```python
from build123d import *

# Parameters (mm, degrees)
CUT_EXTRUDE1_DEPTH = 1.8288


with BuildPart() as part:
    # Sketch1 → Revolve1 (revolve)
    with BuildSketch(Plane.XY, mode=Mode.PRIVATE) as revolve1_sk:
        with BuildLine():
            Line((0, 0), (76.9366, 0))
            Line((76.9366, 0), (76.9366, 2.413))
            Line((76.9366, 2.413), (0.7366, 2.413))
            Line((0.7366, 2.413), (0.7366, 4.5847))
            Line((0.7366, 4.5847), (0.3556, 4.5847))
            ThreePointArc((0.3556, 4.5847), (-0.901703741, 3.66491926), (-1.8288, 2.413))
            Line((-1.8288, 2.413), (-1.8288, 1.8288))
            Line((-1.8288, 1.8288), (0, 0))
        make_face()
    revolve(revolve1_sk.sketch.rotate(Axis((0, 0, 0), (1, 0, 0)), 90), axis=Axis((0, 0, 0), (1, 0, 0)))

    # Sketch2 → Cut-Extrude1 (cut)
    with BuildSketch(Plane.ZY.offset(1.8288)):
        Polygon((1.833087105, 0), (0.916543552, 1.5875), (-0.916543552, 1.5875), (-1.833087105, 0), (-0.916543552, -1.5875), (0.916543552, -1.5875), align=None)
    extrude(amount=-CUT_EXTRUDE1_DEPTH, mode=Mode.SUBTRACT)


solid = part.part
```
Geometry: final body of the model. Coordinates: model frame, mm. A direction names the side the tool comes from. Coordinates: 2 decimals unless noted, no trailing zeros. Order: outer loops, then holes, each group sorted by start corner. A loop starts at its lowest first (then second) coordinate and runs counter-clockwise, first axis right, second up. Notation, with made-up numbers: (-21, 36.5) -> (27, 36.5) arc R28 ccw to (27, 57.5) -> close; hole circle Ø7 at (-10.5, 81). An arc over 180 degrees is marked (long way). Write each question's results on one line, items separated by ' | '. Start each with the question number.
1) Mould query, pull axis Y, two halves, no side actions, for faces 1 (the flat face through (0, 0, 0)), 2 (the flat face through (0.737, 2, -2)), 3 (the cylindrical face through (0.543, 4.476, -0.994)). Classes: released by +Y, released by -Y, zero draft, split by the parting line, or undercut.
2) Cut plane A-A, the plane x = 22.5. Output: boundary loops of the cut face in (y, z).
3) Set-up query: faces 4 (the flat face through (-0.927, -0.783, -1.381)), 5 (the flat face through (-1.829, -2, 0)), 6 (the cylindrical face through (38.303, 1.468, -1.915)). Return all of +Z, -Z, +X, -X, +Y, -Y with unobstructed straight access to the full face (end or side cutting, diameter ignored); none if empty.
4) First-contact query: pin 1 (2 mm diameter, centred on x = 25.5, z = 1.5, fed in from +Y); pin 2 (1.5 mm diameter, centred on x = 52.5, y = 1, fed in from +Z); pin 3 (4 mm diameter, centred on x = 41.5, y = 1, fed in from -Z). Flat tips, straight axial feed; report the tip coordinate or a pass-through.
5) Material intervals for line 1 along X through (y, z) = (0, 1.75); line 2 along Z through (x, y) = (44.5, -0.25), sorted ascending.
Checks:
1) face 1: undercut | face 2: zero draft | face 3: split by the parting line
2) outline: circle Ø4.83 at (0, 0)
3) face 4: -X | face 5: +Z, -Z, -X, +Y, -Y | face 6: +X
4) pin 1: y = 2.36 | pin 2: z = 2.4 | pin 3: z = -2.41
5) line 1: 0 to 76.94 | line 2: -2.4 to 2.4
